Here's how the part is built. I have some questions about the finished solid (model axes, mm). Face numbers are marked on the shaded views. A direction names the side the tool comes from. Give positions to 0.01 mm unless a question says otherwise; leave off trailing zeros. Loops run counter-clockwise (first coordinate to the right, second up) from the corner with the lowest first, then second, coordinate; pieces in that order, holes last. Notation, with made-up numbers: M 24.25,26 L 72.25,26 A18 cw 72.25,45 Z; hole C 66,59 d5. An arc over 180 degrees is marked long. Write item = value, one per line. Start each with the question number.
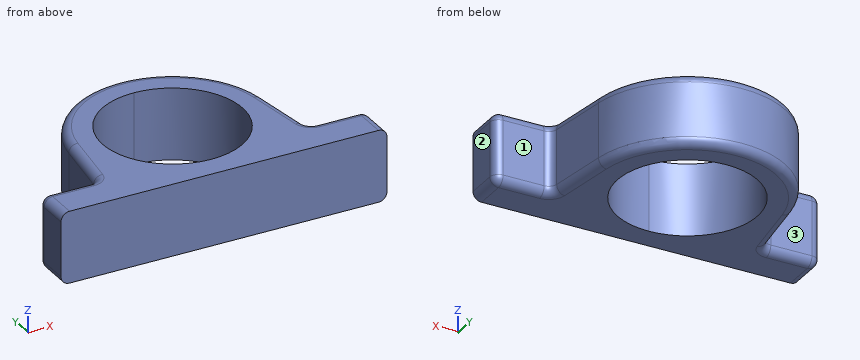
```python
from build123d import *

# Parameters (mm, degrees)
BOSS_EXTRUDE1_DEPTH = 42
FILLET1_R           = 5


with BuildPart() as part:
    # Sketch1 → Boss-Extrude1 (new body)
    with BuildSketch(Plane.XY):
        with BuildLine():
            Line((0, 0), (-95.5, 0))
            Line((-95.5, 0), (-95.5, 23))
            Line((-95.5, 23), (-62.057478344, 23))
            Line((-62.057478344, 23), (-56.445279918, 62.932866755))
            ThreePointArc((-56.445279918, 62.932866755), (-37.395364652, 98.018446073), (0, 112))
            Line((0, 112), (0, 96))
            ThreePointArc((0, 96), (-41, 55), (0, 14))
            Line((0, 14), (0, 0))
        make_face()
    boss_extrude1 = extrude(amount=BOSS_EXTRUDE1_DEPTH)

    # Mirror1: Boss-Extrude1 across plane
    add(boss_extrude1.mirror(Plane(origin=(0, 112, 42), x_dir=(0, 0, 1), z_dir=(-1, 0, 0))))

    # Fillet1
    fillet1_edges = [part.edges().sort_by_distance(p)[0] for p in [
        (0, 112, 0),
        (-95.5, 23, 21),
        (-62.057478344, 23, 21),
        (0, 112, 42),
        (-59.251379131, 42.966433377, 42),
        (95.5, 11.5, 42),
        (-78.778739172, 23, 42),
        (78.778739172, 23, 42),
        (95.5, 23, 21),
        (59.251379131, 42.966433377, 42),
        (62.057478344, 23, 21),
        (59.251379131, 42.966433377, 0),
        (78.778739172, 23, 0),
        (-95.5, 11.5, 42),
        (95.5, 11.5, 0),
        (-95.5, 11.5, 0),
        (-78.778739172, 23, 0),
        (-59.251379131, 42.966433377, 0),
    ]]
    fillet(fillet1_edges, radius=FILLET1_R)


solid = part.part
```
Q1. If we section it at B-B, the plane x = 75.5: List the corners of the cut face in (y, z) for me, then the cut area to 3 significant figures.
Q2. If I drill on line 1 along X through (y, z) = (40.5, 16); line 2 along X through (y, z) = (30, 6); line 3 along Y through (x, z) = (25, 6) (3 decimals), over which ranges is the centre line in solid material (lowest first)?
Q3. Will these pins go through, and if not, where does the flat tip stop? pin 1 (8 mm diameter, centred on y = 59.5, z = 5.5, fed in from +X); pin 2 (10 mm diameter, centred on x = 40.5, z = 23.5, fed in from +Y); pin 3 (8 mm diameter, centred on y = 96.5, z = 29, fed in from -X).
Q4. If we section it at A-A, the plane z = 8: List the corners of the cut face in (x, y) for me.
Q5. On a 3-axis mill with a long thin cutter (end or side, diameter ignored), from which of +Z, -Z, +X, -X, +Y, -Y can I reach the whole of each face in a straight line? I mean the marked faces 1, 2 and 3. Say none if no direction works.
Resolved:
q1.outline = M 0,0 L 18,0 A5 ccw 23,5 L 23,37 A5 ccw 18,42 L 0,42 Z
q1.area = 955 mm²
q2.line_1 = -59.6 to -38.35, 38.35 to 59.6
q2.line_2 = -61.07 to -32.5, 32.5 to 61.07
q2.line_3 = 0 to 22.504, 87.496 to 106.225
q3.pin_1 = 57.49
q3.pin_2 = 99.6
q3.pin_3 = -42.93
q4.outline = M -95.5,0 L 95.5,0 L 95.5,18 A5 ccw 90.5,23 L 66.4,23 A5 cw 61.45,27.3 L 56.45,62.93 A57 ccw -56.45,62.93 L -61.45,27.3 A5 cw -66.4,23 L -90.5,23 A5 ccw -95.5,18 Z; hole C 0,55 d82
q5.face_1 = +Z, -Z, +X, +Y
q5.face_2 = +Z, -Z, +X, +Y, -Y
q5.face_3 = +Z, -Z, -X, +Y
